Autodesk Inventor part; units mm, degrees
ref_plane "YZ Plane" through (0, 0, 0) normal (1, 0, 0) x (0, 1, 0)
ref_plane "XZ Plane" through (0, 0, 0) normal (0, 1, 0) x (-1, 0, 0)
ref_plane "XY Plane" through (0, 0, 0) normal (0, 0, 1) x (1, 0, 0)
sketch "Sketch1" plane through (0, 0, 0) normal (0, 0, 1) x (1, 0, 0)
  line L0 (0.0819, 48.1439) -> (0.0819, -16.0521)
  line L1 (0.0819, 0.0886) -> (20.0819, 0.0886)
  line L2 (20.0819, 0.0886) -> (20.0819, 20.0886)
  line L3 (20.0819, 20.0886) -> (0.0819, 20.0886)
  line L4 (0.0819, 20.0886) -> (0.0819, 0.0886)
  line L5 (0.0819, 0.0886) -> (62.5819, 0.0886)
  line L6 (62.5819, 0.0886) -> (62.5819, -4.9114)
  line L7 (62.5819, -4.9114) -> (0.0819, -4.9114)
  line L8 (0.0819, -4.9114) -> (0.0819, 0.0886)
  line L9 (62.5819, 0.0886) -> (52.5819, 0.0886)
  line L10 (52.5819, 0.0886) -> (52.5819, 20.0886)
  line L11 (52.5819, 20.0886) -> (62.5819, 20.0886)
  line L12 (62.5819, 20.0886) -> (62.5819, 0.0886)
  line L13 (0.0819, -4.9114) -> (20.0819, -4.9114)
  line L14 (20.0819, -4.9114) -> (20.0819, -24.9114)
  line L15 (20.0819, -24.9114) -> (0.0819, -24.9114)
  line L16 (0.0819, -24.9114) -> (0.0819, -4.9114)
  line L17 (52.5819, -4.9114) -> (62.5819, -4.9114)
  line L18 (62.5819, -4.9114) -> (62.5819, -24.9114)
  line L19 (62.5819, -24.9114) -> (52.5819, -24.9114)
  line L20 (52.5819, -24.9114) -> (52.5819, -4.9114)
  dimension "d4" = 62.5
  dimension "d5" = 20
  dimension "d6" = 20
  dimension "d7" = 20
  dimension "d8" = 10
  dimension "d10" = 20
  dimension "d11" = 20
  dimension "d12" = 5
  dimension "d13" = 20
  dimension "d14" = 10
revolve "Revolution2" add sketch "Sketch1" angle 360 about axis through (0.0819, 48.1439, 0) along (0, -1, 0)
fillet "Fillet1" radius 5 2 edges at (-62.4181, 20.0886, 0) (-62.4181, -24.9114, 0)
fillet "Fillet2" radius 5 1 edges at (-19.9181, 0.0886, 0)
fillet "Fillet3" radius 5 1 edges at (-19.9181, -4.9114, 0)
sketch "Sketch2" plane through (0.0819, 20.0886, 0) normal (0, 1, 0) x (1, 0, 0)
  circle A0 centre (-0.0819, 0) radius 18
  dimension "d21" = 36
extrude "Extrusion1" cut sketch "Sketch2" against normal blind 2
sketch "Sketch3" plane through (0.0819, -24.9114, 0) normal (0, -1, 0) x (1, 0, 0)
  circle A0 centre (-0.0819, 0) radius 18
  dimension "d22" = 36
extrude "Extrusion2" cut sketch "Sketch3" against normal blind 2
sketch "Sketch4" plane through (0, 18.0886, 0) normal (0, 1, 0) x (1, 0, 0)
  circle A0 centre (0, 0) radius 7.5
  dimension "d25" = 15
extrude "Extrusion3" cut sketch "Sketch4" against normal through all
properties part number "Wheel" material "Polyethylene, High Density"
Build history of the part. All positions in model axes, mm. A direction names the side the tool comes from. Coordinates: 2 decimals unless noted, no trailing zeros. Write each loop counter-clockwise with the first axis right and the second up, starting at its lowest first coordinate (ties: lowest second). Pieces come first, ordered by that corner, then holes.
1. Drop flat-ended pins along their axis: pin 1 (4 mm diameter, centred on x = 34.5, z = 12, fed in from +Y); pin 2 (9 mm diameter, centred on x = 0, z = 0, fed in from -Y); pin 3 (21.5 mm diameter, centred on x = 0, z = 0, fed in from -Y); pin 4 (11 mm diameter, centred on x = 3, z = 0.5, fed in from +Y). Give the stop position or say it passes through.
Answer block:
pin 1: stops at y = 0.09
pin 2: passes through
pin 3: stops at y = -22.91
pin 4: stops at y = 18.09
2. Pull direction X, two halves, no side cores. Call faces 4 (the flat face through (25, 20.089, -47)), 5 (the cylindrical face through (-13.467, -2.656, -61.014)), 6 (the cylindrical face through (-4.254, -17.516, -19.524)): released by +X, released by -X, zero draft, split by the parting line, or undercut.
Answer block:
face 4: zero draft
face 5: split by the parting line
face 6: undercut
3. 3-axis set-ups, long thin cutter, end or side, ignore diameter. For faces 1 (the cylindrical face through (50.158, -14.771, -15.77)), 2 (the cylindrical face through (50.158, 10.229, -15.77)), 3 (the flat face through (18, 20.089, 3)): which of +Z, -Z, +X, -X, +Y, -Y reach the whole face in a straight line?
Answer block:
face 1: -Y
face 2: +Y
face 3: +Z, -Z, +X, -X, +Y
4. Drill centre lines: probe 1 along Z at (x, y) = (9, 9.5); probe 2 along Z at (x, y) = (0.5, -19); probe 3 along Z at (x, y) = (2, -11). Where is each one in solid material? Low to high.
Answer block:
probe 1: z = -61.86 to -51.74, -17.9 to 17.9, 51.74 to 61.86
probe 2: z = -62.5 to -52.5, -20 to -7.48, 7.48 to 20, 52.5 to 62.5
probe 3: z = -62.47 to -52.46, -19.91 to -7.23, 7.23 to 19.91, 52.46 to 62.47
5. Band-saw the part on B-B, the plane y = -8. Give the cut face in (x, z), and give its area (3 significant figures).
Answer block:
outline: circle Ø125 at (0.08, 0); circle Ø40.76 at (0.08, 0); hole circle Ø105 at (0.08, 0); hole circle Ø15 at (0, 0)
area: 4,740 mm2
6. Band-saw the part on A-A, the plane y = 12. Give the cut face in (x, z), and give its area (3 significant figures).
Answer block:
outline: circle Ø125 at (0.08, 0); circle Ø40 at (0.08, 0); hole circle Ø105 at (0.08, 0); hole circle Ø15 at (0, 0)
area: 4,690 mm2
